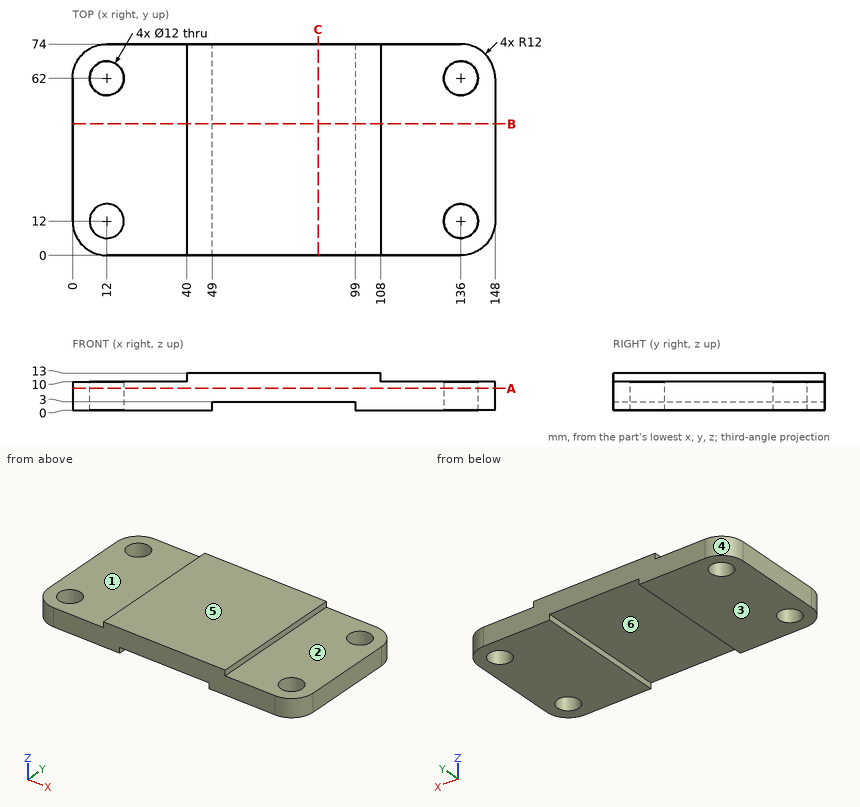
The figure shows three views and two pictorial views of one solid part (mm, origin at its lowest corner). Answer the questions. A direction names the side the tool comes from. Coordinates: 2 decimals unless noted, no trailing zeros. Write each loop counter-clockwise with the first axis right and the second up, starting at its lowest first coordinate (ties: lowest second). Pieces come first, ordered by that corner, then holes.
1. For the marked faces 1, 2 and 3, determine the directions among +Z, -Z, +X, -X, +Y, -Y from which every point of the face is accessible in a straight line to the end or side of a thin tool.
Results list:
face 1: +Z, -X, +Y, -Y
face 2: +Z, +X, +Y, -Y
face 3: -Z, +X, -X, +Y, -Y
2. For a pull along X with two mould halves and no side action, classify the marked faces 4, 5 and 6 as +X half, -X half, draft (parallel to the pull), parting line (faces both ways), or undercut.
Results list:
face 4: -X half
face 5: draft
face 6: undercut
3. Consider line 1 along Y through (x, z) = (12, 8.25); line 2 along X through (y, z) = (62, 6.25); line 3 along X through (y, z) = (54, 1.5). Determine where each line is inside the solid, lowest interval first.
Results list:
line 1: y = 0 to 6, 18 to 56, 68 to 74
line 2: x = 0 to 6, 18 to 130, 142 to 148
line 3: x = 0 to 49, 99 to 148
4. The part is cut by section B-B, the plane y = 46. Write down the section's boundary in (x, z).
Results list:
outline: (0, 0) - (49, 0) - (49, 3) - (99, 3) - (99, 0) - (148, 0) - (148, 10) - (108, 10) - (108, 13) - (40, 13) - (40, 10) - (0, 10) - close
5. Flat-ended cylindrical pins translate along their axes: pin 1 (2 mm diameter, centred on y = 34, z = 2.5, fed in from -X); pin 2 (15 mm diameter, centred on x = 69.5, y = 29, fed in from -Z); pin 3 (8 mm diameter, centred on x = 126.5, y = 30, fed in from +Z); pin 4 (2.5 mm diameter, centred on y = 35.5, z = 12, fed in from +X). Find the tip coordinate at first contact, or state that the pin passes through.
Results list:
pin 1: stops at x = 0
pin 2: stops at z = 3
pin 3: stops at z = 10
pin 4: stops at x = 108
6. The part is cut by section A-A, the plane z = 7.75. Write down the section's boundary in (x, y).
Results list:
outline: (0, 12) arc R12 ccw to (12, 0) - (136, 0) arc R12 ccw to (148, 12) - (148, 62) arc R12 ccw to (136, 74) - (12, 74) arc R12 ccw to (0, 62) - close; hole circle Ø12 at (12, 12); hole circle Ø12 at (12, 62); hole circle Ø12 at (136, 12); hole circle Ø12 at (136, 62)
7. The part is cut by section C-C, the plane x = 86. Write down the section's boundary in (y, z), and give its area (3 significant figures).
Results list:
outline: (0, 3) - (74, 3) - (74, 13) - (0, 13) - close
area: 740 mm2
